The model under review builds one solid part; all positions refer to its coordinate system, in mm. Face numbers are marked on the shaded views. A direction names the side the tool comes from. Round coordinates to 2 decimals unless told otherwise and drop trailing zeros. Order: outer loops, then holes, each group sorted by start corner. A loop starts at its lowest first (then second) coordinate and runs counter-clockwise, first axis right, second up.
1) To check wall thickness, follow L1, parallel to Z at x = 35, y = 78; L2, parallel to Z at x = -14, y = 79; L3, parallel to X at y = 10.5, z = 8.5. State the ranges of each line that lie inside material, in increasing order.
2) Consider section A-A (y = 52). Give the boundary of the cut face in (x, z), then the cut area to 3 significant figures.
3) Machinability: for the marked faces 1 and 2, which of the approach directions +Z, -Z, +X, -X, +Y, -Y give a long, thin tool a straight path to every point of the face, cutting with its end or side? Answer none if there is none.
4) Clearance check with flat-ended pins moving along their axes: P1, Ø5, axis at x = -14.85, z = -9.99, coming from the -Y side; P2, Ø12, axis at y = 8, z = 7.5, coming from the +X side; P3, Ø4.5, axis at y = 78.5, z = -3.5, coming from the -X side. State where each tip first meets the part, or that it passes through.
5) Consider section B-B (y = 30). Give the boundary of the cut face in (x, z).
from build123d import *

# Parameters (mm, degrees)
SKETCH3_W              = 73.802028427
SKETCH3_H              = 33.55074113
BOSS_EXTRUDE1_DEPTH    = 5
BOSS_EXTRUDE2_DEPTH    = 6
CUT_EXTRUDE1_OUTLINE_W = 73.802028427
CUT_EXTRUDE1_OUTLINE_H = 33.55074113
CUT_EXTRUDE1_DEPTH     = 5
SKETCH11_W             = 9.910304241
SKETCH11_H             = 23.835167919
SKETCH11_R             = 2.15
BOSS_EXTRUDE3_DEPTH    = 5.5
BOSS_EXTRUDE3_2_DEPTH  = 5.5
CIRPATTERN3_COUNT      = 3
FILLET3_R              = 5
FILLET4_R              = 20
CUT_EXTRUDE2_DEPTH     = 10
CUT_EXTRUDE3_DEPTH     = 10
FILLET5_R              = 10
FILLET6_R              = 10


# Read off the part's stored shape, not the designer's step: Cut-Extrude1
with BuildPart() as part:
    # Sketch3 → Boss-Extrude1 (new body)
    with BuildSketch(Plane.XY):
        with Locations((2.875089275, 11.32460742)):
            Rectangle(SKETCH3_W, SKETCH3_H)
    extrude(amount=BOSS_EXTRUDE1_DEPTH)

    # Sketch4 → Boss-Extrude2 (add)
    with BuildSketch(Plane.XY.offset(5)):
        with BuildLine():
            Line((-88.363175499, 81.016503161), (88.363175499, 81.016503161))
            ThreePointArc((88.363175499, 81.016503161), (114.343937613, 66.016503161), (114.343937613, 36.016503161))
            Line((114.343937613, 36.016503161), (25.980762114, -117.033006322))
            ThreePointArc((25.980762114, -117.033006322), (0, -132.033006322), (-25.980762114, -117.033006322))
            Line((-25.980762114, -117.033006322), (-114.343937613, 36.016503161))
            ThreePointArc((-114.343937613, 36.016503161), (-114.343937613, 66.016503161), (-88.363175499, 81.016503161))
        make_face()
    extrude(amount=BOSS_EXTRUDE2_DEPTH)

    # Cut-Extrude1 outline → Cut-Extrude1 (cut)
    with BuildSketch(Plane(origin=(0, 0, 5), x_dir=(-1, 0, 0), z_dir=(0, 0, -1))):
        with Locations((-2.875089275, 11.32460742)):
            Rectangle(CUT_EXTRUDE1_OUTLINE_W, CUT_EXTRUDE1_OUTLINE_H)
    extrude(amount=CUT_EXTRUDE1_DEPTH, mode=Mode.SUBTRACT)


with BuildPart() as body_2:
    # Sketch11 → Boss-Extrude3 (new body)
    with BuildSketch(Plane(origin=(0, 81.016503161, 0), x_dir=(1, 0, 0), z_dir=(0, 1, 0))):
        with Locations((-15.667013432, 6.917583959)):
            Rectangle(SKETCH11_W, SKETCH11_H)
        with Locations(Location((-14.850000449, 9.993341923, 0), (0, 0, 180))):
            Circle(SKETCH11_R, mode=Mode.SUBTRACT)
        with Locations(Location((-14.850000449, 0, 0), (0, 0, 180))):
            Circle(SKETCH11_R, mode=Mode.SUBTRACT)
    extrude(amount=-BOSS_EXTRUDE3_DEPTH)


with BuildPart() as body_3:
    # Sketch11 → Boss-Extrude3 2 (new body)
    with BuildSketch(Plane(origin=(0, 81.016503161, 0), x_dir=(1, 0, 0), z_dir=(0, 1, 0))):
        with Locations((35.867012534, 6.917583959)):
            Rectangle(SKETCH11_W, SKETCH11_H)
        with Locations(Location((35.049999551, 9.993341923, 0), (0, 0, 180))):
            Circle(SKETCH11_R, mode=Mode.SUBTRACT)
        with Locations(Location((35.049999551, 0, 0), (0, 0, 180))):
            Circle(SKETCH11_R, mode=Mode.SUBTRACT)
    extrude(amount=-BOSS_EXTRUDE3_2_DEPTH)


with BuildPart() as cirpattern3_1:
    # CirPattern3: pattern copy
    add(body_3.part.rotate(Axis((0, 0, 0), (0, 0, 1)), 1 * 360 / CIRPATTERN3_COUNT))


with BuildPart() as cirpattern3_2:
    # CirPattern3: pattern copy
    add(body_3.part.rotate(Axis((0, 0, 0), (0, 0, 1)), 2 * 360 / CIRPATTERN3_COUNT))


with BuildPart() as cirpattern3_3:
    # CirPattern3: pattern copy
    add(body_2.part.rotate(Axis((0, 0, 0), (0, 0, 1)), 1 * 360 / CIRPATTERN3_COUNT))


with BuildPart() as cirpattern3_4:
    # CirPattern3: pattern copy
    add(body_2.part.rotate(Axis((0, 0, 0), (0, 0, 1)), 2 * 360 / CIRPATTERN3_COUNT))


with BuildPart() as part_1:
    add(part.part)

    # Combine1: union CirPattern3_1, CirPattern3_3, CirPattern3_2, CirPattern3_4, body 3, body 2
    add(cirpattern3_1.part)
    add(cirpattern3_3.part)
    add(cirpattern3_2.part)
    add(cirpattern3_4.part)
    add(body_3.part)
    add(body_2.part)

    # Fillet3
    # the kernel refuses this fillet: 5 mm, written as the material it takes off along each edge
    with BuildSketch(Plane(origin=(30.911860413, 93.516503161, -18.835167919), x_dir=(0, 0, 1), z_dir=(0, -1, 0)), Plane(origin=(-20.622165552, 93.516503161, -18.835167919), x_dir=(0, 0, 1), z_dir=(0, -1, 0)), Plane(origin=(91.298750186, -28.898932331, -18.835167919), x_dir=(0, 0, 1), z_dir=(-0.866025403784445, 0.4999999999999889, 0)), Plane(origin=(65.531737204, -73.528707976, -18.835167919), x_dir=(0, 0, 1), z_dir=(-0.866025403784445, 0.4999999999999889, 0)), Plane(origin=(-96.443597617, -19.987795185, -18.835167919), x_dir=(0, 0, 1), z_dir=(0.8660254037844322, 0.5000000000000114, 0)), Plane(origin=(-70.676584634, -64.61757083, -18.835167919), x_dir=(0, 0, 1), z_dir=(0.8660254037844322, 0.5000000000000114, 0))) as fillet3_piece_1:
        with BuildLine():
            CenterArc((FILLET3_R, -FILLET3_R), FILLET3_R, 90, 90)
            Line((0, -FILLET3_R), (0, 0))
            Line((0, 0), (FILLET3_R, 0))
        make_face()
    extrude(amount=30.5, mode=Mode.SUBTRACT)
    with BuildSketch(Plane(origin=(40.822164654, 93.516503161, -18.835167919), x_dir=(0, 0, 1), z_dir=(0, -1, 0)), Plane(origin=(-10.711861311, 93.516503161, -18.835167919), x_dir=(0, 0, 1), z_dir=(0, -1, 0)), Plane(origin=(86.343598066, -37.481507563, -18.835167919), x_dir=(0, 0, 1), z_dir=(-0.866025403784445, 0.4999999999999889, 0)), Plane(origin=(60.576585084, -82.111283208, -18.835167919), x_dir=(0, 0, 1), z_dir=(-0.866025403784445, 0.4999999999999889, 0)), Plane(origin=(-101.398749737, -11.405219953, -18.835167919), x_dir=(0, 0, 1), z_dir=(0.8660254037844322, 0.5000000000000114, 0)), Plane(origin=(-75.631736755, -56.034995598, -18.835167919), x_dir=(0, 0, 1), z_dir=(0.8660254037844322, 0.5000000000000114, 0))) as fillet3_piece_2:
        with BuildLine():
            CenterArc((FILLET3_R, FILLET3_R), FILLET3_R, 180, 90)
            Line((0, FILLET3_R), (0, 0))
            Line((0, 0), (FILLET3_R, 0))
        make_face()
    extrude(amount=30.5, mode=Mode.SUBTRACT)

    # Fillet4
    # the kernel refuses this fillet: 20 mm, written as the material it adds along each edge
    with BuildSketch(Plane(origin=(80.473432639, -22.648932331, 5), x_dir=(0.4999999999999889, 0.866025403784445, 0), z_dir=(-0.866025403784445, 0.4999999999999889, 0)), Plane(origin=(-59.851267087, -58.36757083, 5), x_dir=(0.5000000000000114, -0.8660254037844322, 0), z_dir=(0.8660254037844322, 0.5000000000000113, 0)), Plane(origin=(-20.622165552, 81.016503161, 5), x_dir=(-1, 0, 0), z_dir=(0, -1, 0))) as fillet4_piece_1:
        with BuildLine():
            CenterArc((19.97284858, 20), FILLET4_R, 182.670565348, 87.329434652)
            Line((-0.005430284, 19.068134335), (-2.00325817, 18.974947769))
            ThreePointArc((-2.00325817, 18.974947769), (-2, 18.835167919), (-2, 0))
            Line((-2, 0), (0, -2))
            Line((0, -2), (19.97284858, -2))
            Line((19.97284858, -2), (19.97284858, 0))
        make_face()
    extrude(amount=5.5)
    with BuildSketch(Plane(origin=(49.751267536, -75.861283208, 5), x_dir=(-0.4999999999999889, -0.8660254037844451, 0), z_dir=(-0.866025403784445, 0.4999999999999889, 0)), Plane(origin=(-90.57343219, -5.155219953, 5), x_dir=(-0.5000000000000113, 0.8660254037844322, 0), z_dir=(0.8660254037844322, 0.5000000000000113, 0)), Plane(origin=(40.822164654, 81.016503161, 5), x_dir=(1, 0, 0), z_dir=(0, -1, 0))) as fillet4_piece_2:
        with BuildLine():
            CenterArc((19.97284858, -20), FILLET4_R, 90, 87.329434652)
            Line((-0.005430284, -19.068134335), (-2.00325817, -18.974947769))
            ThreePointArc((-2.00325817, -18.974947769), (-2, -18.835167919), (-2, 0))
            Line((-2, 0), (0, 2))
            Line((0, 2), (19.97284858, 2))
            Line((19.97284858, 2), (19.97284858, 0))
        make_face()
    extrude(amount=5.5)

    # Sketch13 → Cut-Extrude2 (cut)
    with BuildSketch(Plane.XY.offset(11)):
        with BuildLine():
            Line((-5.215723818, 18.4505975), (-18.576519023, -4.747764108))
            ThreePointArc((-18.576519023, -4.747764108), (-18.570155502, -10.747760733), (-13.370824241, -13.742248075))
            Line((-13.370824241, -13.742248075), (13.39994384, -13.713855334))
            ThreePointArc((13.39994384, -13.713855334), (18.59291158, -10.70834605), (18.586548059, -4.708349425))
            Line((18.586548059, -4.708349425), (5.176575183, 18.461619442))
            ThreePointArc((5.176575183, 18.461619442), (-0.022756078, 21.456106783), (-5.215723818, 18.4505975))
        make_face()
        with BuildLine():
            Line((-44.30857639, 22.581568506), (-33.761718484, 4.313874753))
            ThreePointArc((-33.761718484, 4.313874753), (-31.163642273, 2.813874753), (-28.565566061, 4.313874753))
            Line((-28.565566061, 4.313874753), (-18.018708156, 22.581568506))
            ThreePointArc((-18.018708156, 22.581568506), (-18.018708156, 25.581568506), (-20.616784367, 27.081568506))
            Line((-20.616784367, 27.081568506), (-41.710500179, 27.081568506))
            ThreePointArc((-41.710500179, 27.081568506), (-44.30857639, 25.581568506), (-44.30857639, 22.581568506))
        make_face()
        with BuildLine():
            Line((2.598076211, -49.663137012), (13.144934117, -31.395443259))
            ThreePointArc((13.144934117, -31.395443259), (13.144934117, -28.395443259), (10.546857906, -26.895443259))
            Line((10.546857906, -26.895443259), (-10.546857906, -26.895443259))
            ThreePointArc((-10.546857906, -26.895443259), (-13.144934117, -28.395443259), (-13.144934117, -31.395443259))
            Line((-13.144934117, -31.395443259), (-2.598076211, -49.663137012))
            ThreePointArc((-2.598076211, -49.663137012), (0, -51.163137012), (2.598076211, -49.663137012))
        make_face()
        with BuildLine():
            Line((41.710500179, 27.081568506), (20.616784367, 27.081568506))
            ThreePointArc((20.616784367, 27.081568506), (18.018708156, 25.581568506), (18.018708156, 22.581568506))
            Line((18.018708156, 22.581568506), (28.565566061, 4.313874753))
            ThreePointArc((28.565566061, 4.313874753), (31.163642273, 2.813874753), (33.761718484, 4.313874753))
            Line((33.761718484, 4.313874753), (44.30857639, 22.581568506))
            ThreePointArc((44.30857639, 22.581568506), (44.30857639, 25.581568506), (41.710500179, 27.081568506))
        make_face()
    extrude(amount=-CUT_EXTRUDE2_DEPTH, mode=Mode.SUBTRACT)

    # Sketch14 → Cut-Extrude3 (cut)
    with BuildSketch(Plane(origin=(0, 0, 5), x_dir=(-1, 0, 0), z_dir=(0, 0, -1))):
        with BuildLine():
            Line((-72.464929389, 81.016503161), (-106.394814558, 22.248218154))
            Line((-106.394814558, 22.248218154), (-114.343937613, 36.016503161))
            ThreePointArc((-114.343937613, 36.016503161), (-114.343937613, 66.016503161), (-88.363175499, 81.016503161))
            Line((-88.363175499, 81.016503161), (-72.464929389, 81.016503161))
        make_face()
        with BuildLine():
            Line((106.394814558, 22.248218154), (72.464929389, 81.016503161))
            Line((72.464929389, 81.016503161), (88.363175499, 81.016503161))
            ThreePointArc((88.363175499, 81.016503161), (114.343937613, 66.016503161), (114.343937613, 36.016503161))
            Line((114.343937613, 36.016503161), (106.394814558, 22.248218154))
        make_face()
        with BuildLine():
            Line((-33.929885169, -103.264721315), (33.929885169, -103.264721315))
            Line((33.929885169, -103.264721315), (25.980762114, -117.033006322))
            ThreePointArc((25.980762114, -117.033006322), (0, -132.033006322), (-25.980762114, -117.033006322))
            Line((-25.980762114, -117.033006322), (-33.929885169, -103.264721315))
        make_face()
    extrude(amount=-CUT_EXTRUDE3_DEPTH, mode=Mode.SUBTRACT)

    # Fillet5
    fillet5_edges = [part_1.edges().sort_by_distance(p)[0] for p in [
        (72.464929389, 81.016503161, 8),
    ]]
    fillet(fillet5_edges, radius=FILLET5_R)

    # Fillet6
    fillet6_edges = [part_1.edges().sort_by_distance(p)[0] for p in [
        (106.394814558, 22.248218154, 8),
        (-72.464929389, 81.016503161, 8),
        (-106.394814558, 22.248218154, 8),
        (-33.929885169, -103.264721315, 8),
        (33.929885169, -103.264721315, 8),
    ]]
    fillet(fillet6_edges, radius=FILLET6_R)


solid = part_1.part
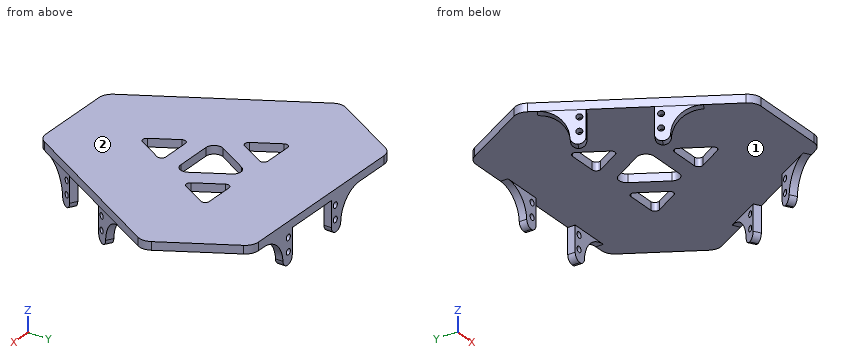
Answer below:
1. L1: z = -18.75 to -12.14, -7.84 to -2.15, 2.15 to 11
1. L2: z = -18.53 to -11.97, -8.02 to -1.97, 1.97 to 11
1. L3: x = -99.61 to -37.33, -24.99 to -9.79, 9.78 to 24.99, 37.33 to 99.61
2. outline: (-89.22, 5) - (89.22, 5) - (89.22, 11) - (-89.22, 11) - close
2. area: 1,070 mm2
3. face 1: -Z
3. face 2: +Z, +X, -X, +Y, -Y
4. P1: stops at y = 75.52
4. P2: stops at x = 101.63
4. P3: stops at x = -26.07
5. outline: (-101.92, 5) - (101.92, 5) - (101.92, 11) - (-101.92, 11) - close
